```python
from build123d import *

# Parameters (mm, degrees)
F0_W     = 470
F0_H     = 250
F1_DEPTH = 5
F2_R     = 1
F3_D     = 50


with BuildPart() as f1:
    # F0 (on Top) → F1 (new body)
    with BuildSketch(Plane.XY):
        Rectangle(F0_W, F0_H)
        with BuildLine():
            ThreePointArc((-193.731551, 10), (-185, 18.731551), (-176.268449, 10))
            Line((-176.268449, 10), (-176.268449, -10))
            ThreePointArc((-176.268449, -10), (-185, -18.731551), (-193.731551, -10))
            Line((-193.731551, -10), (-193.731551, 10))
        make_face(mode=Mode.SUBTRACT)
    extrude(amount=F1_DEPTH)

    # F2
    f2_edges = [f1.edges().sort_by_distance(p)[0] for p in [
        (-235, -125, 2.5),
        (235, -125, 2.5),
        (0, -125, 0),
        (0, -125, 5),
        (235, 125, 2.5),
        (235, 0, 0),
        (235, 0, 5),
        (-235, 125, 2.5),
        (-235, 0, 0),
        (-235, 0, 5),
        (0, 125, 0),
        (0, 125, 5),
    ]]
    fillet(f2_edges, radius=F2_R)

    # F3 (through all)
    with Locations(Plane(origin=(0, 0, 0), x_dir=(1, 0, 0), z_dir=(0, 0, -1))):
        with Locations((-145, 62.5), (-145, -62.5), (-50, -62.5), (-50, 62.5), (45, 62.5), (45, -62.5)):
            Hole(F3_D / 2)


solid = f1.part
```
Could you check a few things on this model? Use its own coordinates, in mm. A direction names the side the tool comes from. Coordinates: 2 decimals unless noted, no trailing zeros. Loops run counter-clockwise (first coordinate to the right, second up) from the corner with the lowest first, then second, coordinate; pieces in that order, holes last.
1) Imagine slicing it at C-C (y = 53.5). List the corners of the cut face in (x, z) for me.
Reported:
outline: (-235, 1) arc R1 ccw to (-234, 0) - (-168.32, 0) - (-168.32, 5) - (-234, 5) arc R1 ccw to (-235, 4) - close; (-121.68, 0) - (-73.32, 0) - (-73.32, 5) - (-121.68, 5) - close; (-26.68, 0) - (21.68, 0) - (21.68, 5) - (-26.68, 5) - close; (68.32, 0) - (234, 0) arc R1 ccw to (235, 1) - (235, 4) arc R1 ccw to (234, 5) - (68.32, 5) - close
2) Imagine slicing it at B-B (z = 2.2). List the corners of the cut face in (x, y) for me.
Reported:
outline: (-235, -124) arc R1 ccw to (-234, -125) - (234, -125) arc R1 ccw to (235, -124) - (235, 124) arc R1 ccw to (234, 125) - (-234, 125) arc R1 ccw to (-235, 124) - close; hole (-193.73, -10) arc R8.73 ccw to (-176.27, -10) - (-176.27, 10) arc R8.73 ccw to (-193.73, 10) - close; hole circle Ø50 at (-145, -62.5); hole circle Ø50 at (-145, 62.5); hole circle Ø50 at (-50, -62.5); hole circle Ø50 at (-50, 62.5); hole circle Ø50 at (45, -62.5); hole circle Ø50 at (45, 62.5)
3) Imagine slicing it at D-D (y = -62.5). List the corners of the cut face in (x, z) for me.
Reported:
outline: (-235, 1) arc R1 ccw to (-234, 0) - (-170, 0) - (-170, 5) - (-234, 5) arc R1 ccw to (-235, 4) - close; (-120, 0) - (-75, 0) - (-75, 5) - (-120, 5) - close; (-25, 0) - (20, 0) - (20, 5) - (-25, 5) - close; (70, 0) - (234, 0) arc R1 ccw to (235, 1) - (235, 4) arc R1 ccw to (234, 5) - (70, 5) - close
4) Please list where these lines run through material, in increasing order: line 1 along Y through (x, z) = (-51.5, 3.1); line 2 along X through (y, z) = (-1, 4.1); line 3 along Y through (x, z) = (-140, 1.65).
Reported:
line 1: y = -125 to -87.45, -37.55 to 37.55, 87.45 to 125
line 2: x = -234.99 to -193.73, -176.27 to 234.99
line 3: y = -125 to -86.99, -38.01 to 38.01, 86.99 to 125
5) Thinking about a two-plate mould opening in Y: for faces 1 (the face through (-126.574, -79.396, 2.535)), 2 (the face through (-3, 2, 5)), which applies, released by +Y, released by -Y, zero draft, split by the parting line, or undercut?
Reported:
face 1: undercut
face 2: zero draft
6) Imagine slicing it at A-A (x = -145). List the corners of the cut face in (y, z) for me.
Reported:
outline: (-125, 1) arc R1 ccw to (-124, 0) - (-87.5, 0) - (-87.5, 5) - (-124, 5) arc R1 ccw to (-125, 4) - close; (-37.5, 0) - (37.5, 0) - (37.5, 5) - (-37.5, 5) - close; (87.5, 0) - (124, 0) arc R1 ccw to (125, 1) - (125, 4) arc R1 ccw to (124, 5) - (87.5, 5) - close
7) Which directions (+Z, -Z, +X, -X, +Y, -Y) give clear straight access to the entire face, cutting with the end or side of a thin tool? Please do faces 3 (the face through (-184.81, -18.73, 2.46)), 4 (the face through (-3, 2, 0)).
Reported:
face 3: +Z, -Z
face 4: -Z, +X, -X, +Y, -Y
